from build123d import *

# Parameters (mm, degrees)
SKETCH1_R           = 70
SKETCH1_R_2         = 30
BOSS_EXTRUDE1_DEPTH = 40
SKETCH2_R           = 79
SKETCH2_R_2         = 30
BOSS_EXTRUDE2_DEPTH = 10
CUT_EXTRUDE1_DEPTH  = 150.939987995


with BuildPart() as part:
    # Sketch1 → Boss-Extrude1 (new, symmetric)
    with BuildSketch(Plane.XY):
        Circle(SKETCH1_R)
        Circle(SKETCH1_R_2, mode=Mode.SUBTRACT)
    extrude(amount=BOSS_EXTRUDE1_DEPTH, both=True)

    # Sketch2 → Boss-Extrude2 (add)
    with BuildSketch(Plane.XY.offset(40)):
        Circle(SKETCH2_R)
        Circle(SKETCH2_R_2, mode=Mode.SUBTRACT)
    boss_extrude2 = extrude(amount=BOSS_EXTRUDE2_DEPTH)

    # Mirror1: Boss-Extrude2 across plane
    add(boss_extrude2.mirror(Plane.XY))

    # Sketch3 → Cut-Extrude1 (cut, through all)
    with BuildSketch(Plane.XY.offset(50)):
        with BuildLine():
            Line((9, 16.370254424), (9, 33.20180718))
            ThreePointArc((9, 33.20180718), (0, 34.4), (-9, 33.20180718))
            Line((-9, 33.20180718), (-9, 16.370254424))
            Line((-9, 16.370254424), (9, 16.370254424))
        make_face()
    extrude(amount=-CUT_EXTRUDE1_DEPTH, mode=Mode.SUBTRACT)


solid = part.part
Can you work these out from the model? Positions are in its coordinate system, mm. A direction names the side the tool comes from. Coordinates: 2 decimals unless noted, no trailing zeros. Order: outer loops, then holes, each group sorted by start corner. A loop starts at its lowest first (then second) coordinate and runs counter-clockwise, first axis right, second up. Notation, with made-up numbers: M 47.5,-38.5 L 88.5,-38.5 A22 cw 88.5,-30.5 Z; hole C 49,85 d11. An arc over 180 degrees is marked long. Write item = value, one per line.
(1) Suppose I cut it at B-B on y = 0. Please give me the cut outline in (x, z), plus the area to 3 significant figures.
Results are:
outline = M -79,-50 L -30,-50 L -30,50 L -79,50 L -79,40 L -70,40 L -70,-40 L -79,-40 Z; M 30,-50 L 79,-50 L 79,-40 L 70,-40 L 70,40 L 79,40 L 79,50 L 30,50 Z
area = 8,360 mm2
(2) Suppose I cut it at C-C on z = -15. Please give me the cut outline in (x, y), plus the area to 3 significant figures.
Results are:
outline = C 0,0 d140; hole M -9,28.62 A30 ccw long 9,28.62 L 9,33.2 A34.4 ccw -9,33.2 Z
area = 12,500 mm2
(3) For faces 4 (the face through (34, 1, -50)), 5 (the face through (-9, 31, 1)), 6 (the face through (-6, -70, -40)), which set-ups out of +Z, -Z, +X, -X, +Y, -Y let a thin tool reach every point of the face, with its end or its side?
Results are:
face_4 = -Z, +X, -X, +Y, -Y
face_5 = +Z, -Z
face_6 = none
(4) Suppose I cut it at A-A on x = 0. Please give me the cut outline in (y, z), plus the area to 3 significant figures.
Results are:
outline = M -79,-50 L -30,-50 L -30,50 L -79,50 L -79,40 L -70,40 L -70,-40 L -79,-40 Z; M 34.4,-50 L 79,-50 L 79,-40 L 70,-40 L 70,40 L 79,40 L 79,50 L 34.4,50 Z
area = 7,920 mm2
(5) Suppose I cut it at D-D on y = -44.5. Please give me the cut outline in (x, z), plus the area to 3 significant figures.
Results are:
outline = M -65.27,-50 L 65.27,-50 L 65.27,-40 L 54.03,-40 L 54.03,40 L 65.27,40 L 65.27,50 L -65.27,50 L -65.27,40 L -54.03,40 L -54.03,-40 L -65.27,-40 Z
area = 11,300 mm2
(6) For pin 1 Ø3.5 at (y, z) = (30, -9) entering from +X; pin 2 Ø1 at (y, z) = (-18, 29.5) entering from +X; pin 3 Ø5 at (y, z) = (59.5, -38.5) entering from -X, each with a flat end and sliding along its axis, tell me the tip position at first contact or that it passes through.
Results are:
pin_1 = 64.05
pin_2 = 67.78
pin_3 = -54.17
(7) If we mould it in two halves opening along Y, with no side actions, what happens to faces 1 (the face through (-6, -70, 40)), 2 (the face through (-55.55, -42.594, 0.56)), 3 (the face through (9, 31, 1))? For each: pulls with the +Y half, pulls with the -Y half, needs draft (parallel to the pull), parting line crosses it, or undercut.
Results are:
face_1 = needs draft
face_2 = parting line crosses it
face_3 = undercut
(8) I need wall thicknesses on line 1 along Z through (x, y) = (53, -56.5); line 2 along Y through (x, z) = (0, -16.5); line 3 along Y through (x, z) = (-3.5, 4). Which ranges of each line are inside material? Lowest first, please. Write a range as [from, to].
Results are:
line_1 = [-50, -40], [40, 50]
line_2 = [-70, -30], [34.4, 70]
line_3 = [-69.91, -29.8], [34.22, 69.91]
